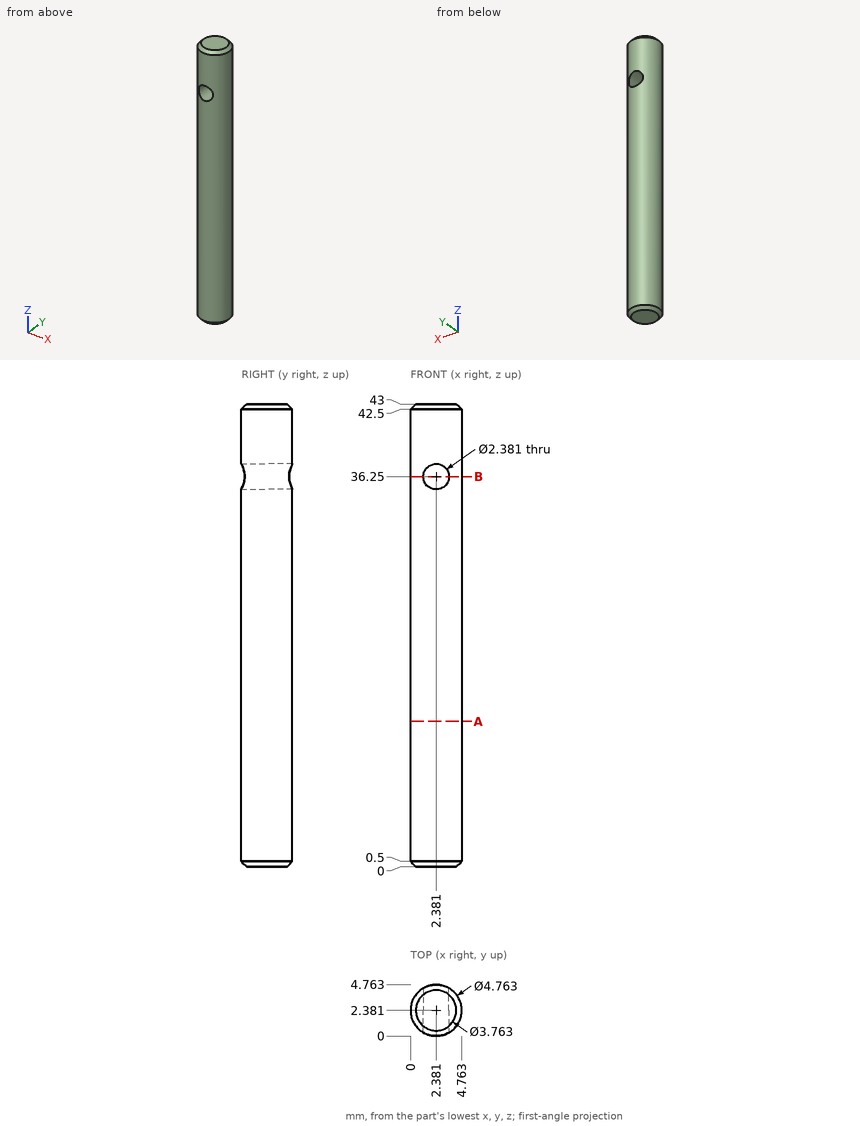
Design review of the part shown in the three views and the two pictorial views. Dimensions are in mm from the part's minimum x, y and z. Round coordinates to 2 decimals unless told otherwise and drop trailing zeros. Loops run counter-clockwise (first coordinate to the right, second up) from the corner with the lowest first, then second, coordinate; pieces in that order, holes last.
Q1. Add section A-A on z = 13.5. Write out the cut boundary in (x, y).
Result sheet:
outline: circle Ø4.76 at (2.38, 2.38)
Q2. Insertion check: pin 1 Ø2 at (x, z) = (3.5, 23) entering from -Y; pin 2 Ø1.5 at (y, z) = (0.5, 32) entering from +X. Each pin has a flat end and moves straight along its axis. Give the tip position at first contact, or say it passes through.
Result sheet:
pin 1: stops at y = 0
pin 2: stops at x = 4.48
Q3. Add section B-B on z = 36.25. Write out the cut boundary in (x, y).
Result sheet:
outline: (1.19, 0.32) - (1.19, 4.44) arc R2.38 ccw to start; (3.57, 0.32) arc R2.38 ccw to (3.57, 4.44) - close
Q4. To check wall thickness, follow line 1 along Z through (x, y) = (3.3, 4.05) (1 decimal); line 2 along Z through (x, y) = (1.8, 0.9); line 3 along X through (y, z) = (0.75, 36.25) (1 decimal). State the ranges of each line that lie inside material, in increasing order.
Result sheet:
line 1: z = 0 to 35.5, 37 to 43
line 2: z = 0 to 35.21, 37.29 to 43
line 3: x = 0.6 to 1.2, 3.6 to 4.1
